Here's how the part is built. I have some questions about the finished solid (model axes, mm). Face numbers are marked on the shaded views. A direction names the side the tool comes from. Give positions to 0.01 mm unless a question says otherwise; leave off trailing zeros. Write each loop counter-clockwise with the first axis right and the second up, starting at its lowest first coordinate (ties: lowest second). Pieces come first, ordered by that corner, then holes. Notation, with made-up numbers: (5, -27.5) -> (10, -27.5) arc R6 cw to (10, -19.5) -> close; hole circle Ø8 at (33.25, -31). An arc over 180 degrees is marked (long way). Use one line per item in the form item = value.
```python
from build123d import *

# Parameters (mm, degrees)
F0_W     = 304.8
F0_H     = 203.2
F1_DEPTH = 203.2
F2_R     = 17.4625
F2_R_2   = 15.875
F3_DEPTH = 254
F4_R     = 15.875
F4_R_2   = 12.7
F5_DEPTH = 50.8


with BuildPart() as f1:
    # F0 (on Front) → F1 (new body)
    with BuildSketch(Plane.XZ):
        with Locations((152.4, 101.6)):
            Rectangle(F0_W, F0_H)
    extrude(amount=F1_DEPTH)

    # F2 (on face) → F3 (join)
    with BuildSketch(Plane.YZ.offset(304.8)):
        with Locations((-101.6, 101.6)):
            Circle(F2_R)
        with Locations((-101.6, 101.6)):
            Circle(F2_R_2, mode=Mode.SUBTRACT)
    extrude(amount=F3_DEPTH)

    # F4 (on face) → F5 (join)
    with BuildSketch(Plane.XY.offset(203.2)):
        with Locations((228.6, -101.6)):
            Circle(F4_R)
        with Locations((228.6, -101.6)):
            Circle(F4_R_2, mode=Mode.SUBTRACT)
    extrude(amount=F5_DEPTH)


solid = f1.part
```
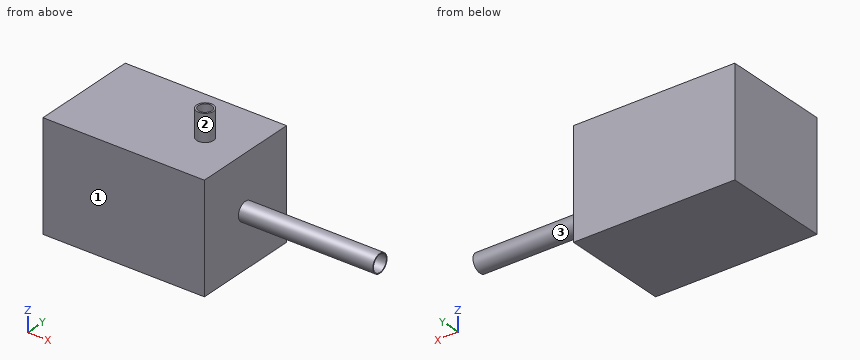
Q1. I want a section at A-A, the plane z = 101.6. Write out the boundary of the cut face in (x, y) (1 decimal).
Result set:
outline = (0, -203.2) -> (304.8, -203.2) -> (304.8, -119.1) -> (558.8, -119.1) -> (558.8, -117.5) -> (304.8, -117.5) -> (304.8, -85.7) -> (558.8, -85.7) -> (558.8, -84.1) -> (304.8, -84.1) -> (304.8, 0) -> (0, 0) -> close
Q2. Will these pins go through, and if not, where does the flat tip stop? pin 1 Ø3 at (x, z) = (358, 108) entering from +Y; pin 2 Ø10 at (y, z) = (-77, 140) entering from +X.
Result set:
pin_1 = -84.84
pin_2 = 304.8
Q3. If I drill on line 1 along Z through (x, y) = (465.5, -101.6) (1 decimal); line 2 along Y through (x, z) = (369, 101); line 3 along X through (y, z) = (-193.5, 103), over which ranges is the centre line in solid material (lowest first)? Write a range as from..to.
Result set:
line_1 = 84.1..85.7, 117.5..119.1
line_2 = -119.05..-117.46, -85.74..-84.15
line_3 = 0..304.8
Q4. I want a section at C-C, the plane y = -127. Write out the boundary of the cut face in (x, z).
Result set:
outline = (0, 0) -> (304.8, 0) -> (304.8, 203.2) -> (0, 203.2) -> close
Q5. Which directions (+Z, -Z, +X, -X, +Y, -Y) give clear straight access to the entire face, cutting with the end or side of a thin tool? Please do the marked faces 1, 2 and 3.
Result set:
face_1 = +Z, -Z, +X, -X, -Y
face_2 = +Z
face_3 = +X
Q6. I want a section at B-B, the plane x = 228.6. Write out the boundary of the cut face in (y, z) (3 decimals).
Result set:
outline = (-203.2, 0) -> (0, 0) -> (0, 203.2) -> (-85.725, 203.2) -> (-85.725, 254) -> (-88.9, 254) -> (-88.9, 203.2) -> (-114.3, 203.2) -> (-114.3, 254) -> (-117.475, 254) -> (-117.475, 203.2) -> (-203.2, 203.2) -> close
Q7. I want a section at D-D, the plane z = 219. Write out the boundary of the cut face in (x, y) (3 decimals), and give its area (3 significant figures).
Result set:
outline = circle Ø31.75 at (228.6, -101.6); hole circle Ø25.4 at (228.6, -101.6)
area = 285 mm2
